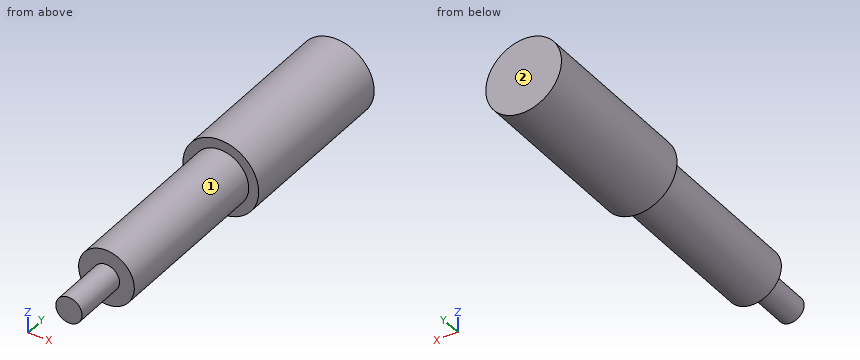
from build123d import *

# Parameters (mm, degrees)
SKETCH2_W   = 12.720955
SKETCH2_H   = 33.02
SKETCH2_W_2 = 5.999999938
SKETCH2_H_2 = 25.4


with BuildPart() as part:
    # Sketch2 → Revolve1 (revolve)
    with BuildSketch(Plane.XY, mode=Mode.PRIVATE) as revolve1_sk:
        with Locations((6.3604775, 86.36)):
            Rectangle(SKETCH2_W, SKETCH2_H)
        Polygon((0, 181.102), (0, 102.87), (12.720955, 102.87), (17.272, 102.87), (17.272, 181.102), align=None)
        Polygon((0, 69.85), (0, 25.4), (5.999999938, 25.4), (12.720955, 25.4), (12.720955, 69.85), align=None)
        with Locations((2.999999969, 12.7)):
            Rectangle(SKETCH2_W_2, SKETCH2_H_2)
    revolve(revolve1_sk.sketch.rotate(Axis((0, 0, 0), (0, 1, 0)), 90), axis=Axis((0, 0, 0), (0, 1, 0)))


solid = part.part
Check sheet for the modelled part. Datum: model origin and axes. Units: mm. Face numbers are marked on the shaded views. A direction names the side the tool comes from. Give positions to 0.01 mm unless a question says otherwise; leave off trailing zeros. Loops run counter-clockwise (first coordinate to the right, second up) from the corner with the lowest first, then second, coordinate; pieces in that order, holes last. Notation, with made-up numbers: M 2,68 L 17,68 A20 ccw 17,98 Z; hole C -1,39 d8. An arc over 180 degrees is marked long. Return JSON: item names as keys, results as strings. Group by question number.
1. Go/stop test with flat-tipped pins: pin 1 (1.5 mm diameter, centred on y = 28.5, z = -9.5, fed in from +X); pin 2 (2 mm diameter, centred on y = 120.5, z = -13.5, fed in from -X); pin 3 (5 mm diameter, centred on x = 6, y = 144.5, fed in from +Z). Record where each tip stops, or that it passes through.
2. Cross-section at C-C on y = 82.5. Record the boundary of the cut face in (x, z), plus the area to 3 significant figures.
3. Cross-section at D-D on x = 8. Record the boundary of the cut face in (y, z), plus the area to 3 significant figures.
4. Tool access check on the marked faces 1 and 2. Record the directions out of +Z, -Z, +X, -X, +Y, -Y that give a thin tool (end or side, any length) a straight path to the whole face; none if there is none.
5. Cross-section at A-A on x = 0. Record the boundary of the cut face in (y, z).
6. Cross-section at B-B on z = 0. Record the boundary of the cut face in (x, y).
7. Thickness scan on L1, parallel to Y at x = 15, z = 3.5; L2, parallel to Y at x = 7, z = -1.5; L3, parallel to Z at x = -6.5, y = 113. Record the ranges inside material, lowest first.
Return value:
{
 "1": {"pin 1": "x = 9.23", "pin 2": "x = -11.92", "pin 3": "z = 16.91"},
 "2": {"outline": "C 0,0 d25.44", "area": "508 mm^2"},
 "3": {"outline": "M 25.4,-9.89 L 102.87,-9.89 L 102.87,-15.31 L 181.1,-15.31 L 181.1,15.31 L 102.87,15.31 L 102.87,9.89 L 25.4,9.89 Z", "area": "3,930 mm^2"},
 "4": {"face 1": "-Y", "face 2": "+Z, -Z, +X, -X, +Y"},
 "5": {"outline": "M 0,-6 L 25.4,-6 L 25.4,-12.72 L 102.87,-12.72 L 102.87,-17.27 L 181.1,-17.27 L 181.1,17.27 L 102.87,17.27 L 102.87,12.72 L 25.4,12.72 L 25.4,6 L 0,6 Z"},
 "6": {"outline": "M -17.27,102.87 L -12.72,102.87 L -12.72,25.4 L -6,25.4 L -6,0 L 6,0 L 6,25.4 L 12.72,25.4 L 12.72,102.87 L 17.27,102.87 L 17.27,181.1 L -17.27,181.1 Z"},
 "7": {"L1": "102.87 to 181.1", "L2": "25.4 to 181.1", "L3": "-16 to 16"}
}
